Can you work these out from the model? Positions are in its coordinate system, mm. Coordinates: 2 decimals unless noted, no trailing zeros. Loops run counter-clockwise (first coordinate to the right, second up) from the corner with the lowest first, then second, coordinate; pieces in that order, holes last.
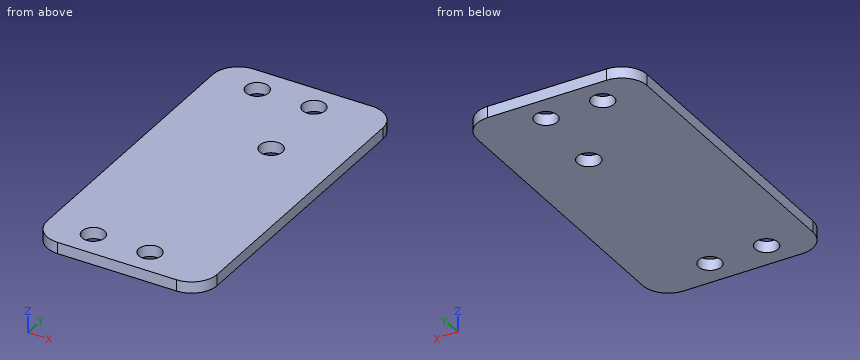
```python
from build123d import *

# Parameters (mm, degrees)
SKETCH1_W           = 30
SKETCH1_H           = 58
SKETCH1_R           = 2
SKETCH1_R_2         = 2.01
BOSS_EXTRUDE1_DEPTH = 2
FILLET1_R           = 4.5


with BuildPart() as part:
    # Sketch1 → Boss-Extrude1 (new body)
    with BuildSketch(Plane.XY):
        Rectangle(SKETCH1_W, SKETCH1_H)
        with Locations((3, 24.25)):
            Circle(SKETCH1_R, mode=Mode.SUBTRACT)
        with Locations((-7, 24.25)):
            Circle(SKETCH1_R, mode=Mode.SUBTRACT)
        with Locations((-7, -24.25)):
            Circle(SKETCH1_R, mode=Mode.SUBTRACT)
        with Locations((3, -24.25)):
            Circle(SKETCH1_R, mode=Mode.SUBTRACT)
        with Locations((3.5, 10.75)):
            Circle(SKETCH1_R_2, mode=Mode.SUBTRACT)
    extrude(amount=BOSS_EXTRUDE1_DEPTH)

    # Fillet1
    fillet1_edges = [part.edges().sort_by_distance(p)[0] for p in [
        (-15, 29, 1),
        (15, 29, 1),
        (15, -29, 1),
        (-15, -29, 1),
    ]]
    fillet(fillet1_edges, radius=FILLET1_R)


solid = part.part
```
(1) I want a section at D-D on x = 3.5. Write out the boundary of the cut face in (y, z).
Check values:
outline: (-29, 0) - (-26.19, 0) - (-26.19, 2) - (-29, 2) - close; (-22.31, 0) - (8.74, 0) - (8.74, 2) - (-22.31, 2) - close; (12.76, 0) - (22.31, 0) - (22.31, 2) - (12.76, 2) - close; (26.19, 0) - (29, 0) - (29, 2) - (26.19, 2) - close
(2) I'm going to push a flat-ended pin straight in: pin 1 (3.5 mm diameter, centred on x = 3, y = 24.25, fed in from -Z). Where does the tip first touch, or does it pass through?
Check values:
pin 1: passes through
(3) I want a section at B-B on y = 10.75. Write out the boundary of the cut face in (x, z), then the cut area to 3 significant figures.
Check values:
outline: (-15, 0) - (1.49, 0) - (1.49, 2) - (-15, 2) - close; (5.51, 0) - (15, 0) - (15, 2) - (5.51, 2) - close
area: 52.0 mm2
(4) I want a section at A-A on x = -7. Write out the boundary of the cut face in (y, z).
Check values:
outline: (-29, 0) - (-26.25, 0) - (-26.25, 2) - (-29, 2) - close; (-22.25, 0) - (22.25, 0) - (22.25, 2) - (-22.25, 2) - close; (26.25, 0) - (29, 0) - (29, 2) - (26.25, 2) - close
(5) I want a section at C-C on z = 1.45. Write out the boundary of the cut face in (x, y), then the cut area to 3 significant figures.
Check values:
outline: (-15, -24.5) arc R4.5 ccw to (-10.5, -29) - (10.5, -29) arc R4.5 ccw to (15, -24.5) - (15, 24.5) arc R4.5 ccw to (10.5, 29) - (-10.5, 29) arc R4.5 ccw to (-15, 24.5) - close; hole circle Ø4 at (-7, -24.25); hole circle Ø4 at (-7, 24.25); hole circle Ø4 at (3, -24.25); hole circle Ø4 at (3, 24.25); hole circle Ø4.02 at (3.5, 10.75)
area: 1,660 mm2
(6) If I drill on probe 1 along Y at (x, z) = (-7, 1.35); probe 2 along Y at (x, z) = (-7.75, 1.6); probe 3 along X at (y, z) = (-25, 0.4), over which ranges is the centre line in solid material (lowest first)?
Check values:
probe 1: y = -29 to -26.25, -22.25 to 22.25, 26.25 to 29
probe 2: y = -29 to -26.1, -22.4 to 22.4, 26.1 to 29
probe 3: x = -14.97 to -8.85, -5.15 to 1.15, 4.85 to 14.97
